Autodesk Inventor part; units mm, degrees
ref_plane "YZ Plane" through (0, 0, 0) normal (1, 0, 0) x (0, 1, 0)
ref_plane "XZ Plane" through (0, 0, 0) normal (0, 1, 0) x (-1, 0, 0)
ref_plane "XY Plane" through (0, 0, 0) normal (0, 0, 1) x (1, 0, 0)
sketch "Sketch1" plane through (0, 0, 0) normal (0, 0, 1) x (1, 0, 0)
  circle A0 centre (0, 0) radius 15
  dimension "d0" = 30
extrude "Extrusion1" add sketch "Sketch1" along normal blind 50
sketch "Sketch2" plane through (0, 0, 50) normal (0, 0, 1) x (1, 0, 0)
  point P0 (0, 0)
sketch "Sketch3" plane through (0, 0, 0) normal (1, 0, 0) x (0, 1, 0)
  arc A0 (-2.5, 0) -> (2.5, 0) centre (0, 0) ccw
  arc A1 (-3, 0) -> (3, 0) centre (0, 0) ccw
  line L0 (-15, 0) -> (15, 0)
  line L1 (3, 0) -> (2.5, 0)
  line L2 (-2.5, 0) -> (-3, 0)
  dimension "d3" = 5
  dimension "d4" = 6
extrude "Extrusion2" add sketch "Sketch3" along normal mid plane 5 contours A0 L0 A1
fillet "Fillet1" radius 2 2 edges at (-15, 0, 50) (-15, 0, 0)
sketch "Sketch4" plane through (0, 0, 0) normal (0, 0, -1) x (-1, 0, 0)
  circle A0 centre (0, 0) radius 0.5
  dimension "d8" = 1
extrude "Extrusion3" add sketch "Sketch4" along normal blind 10
properties part number "weigth"
Check sheet for the modelled part. Datum: model origin and axes. Units: mm. Give positions to 0.01 mm unless a question says otherwise; leave off trailing zeros. Write each loop counter-clockwise with the first axis right and the second up, starting at its lowest first coordinate (ties: lowest second). Pieces come first, ordered by that corner, then holes. Notation, with made-up numbers: (1, -39) -> (6, -39) arc R32 cw to (6, -5) -> close; hole circle Ø6 at (89.5, -4.5). An arc over 180 degrees is marked (long way). One line per item, written item: value. Start each with the question number.
Item 1: Material ranges on probe 1 along Z at (x, y) = (10.25, -7); probe 2 along X at (y, z) = (0, -4); probe 3 along X at (y, z) = (-0.5, 14), recorded low to high. Write a range as from..to.
Item 2: Section check A-A on z = -6. Record the cut outline in (x, y), then the cut area to 3 significant figures.
Item 3: Gauge pin test, flat ends, axial feed: pin 1 (5 mm diameter, centred on y = 11.5, z = 11, fed in from +X); pin 2 (1.5 mm diameter, centred on x = -8, y = -1, fed in from -Z); pin 3 (10 mm diameter, centred on y = -6.5, z = 20, fed in from -X). Record the tip position at first contact, or that the pin passes through.
Item 4: Section check B-B on z = 33. Record the cut outline in (x, y), then the cut area to 3 significant figures.
Results list:
1. probe 1: 0..50
1. probe 2: -0.5..0.5
1. probe 3: -14.99..14.99
2. outline: circle Ø1 at (0, 0)
2. area: 0.785 mm²
3. pin 1: x = 12
3. pin 2: z = 0
3. pin 3: x = -14.92
4. outline: circle Ø30 at (0, 0)
4. area: 707 mm²
